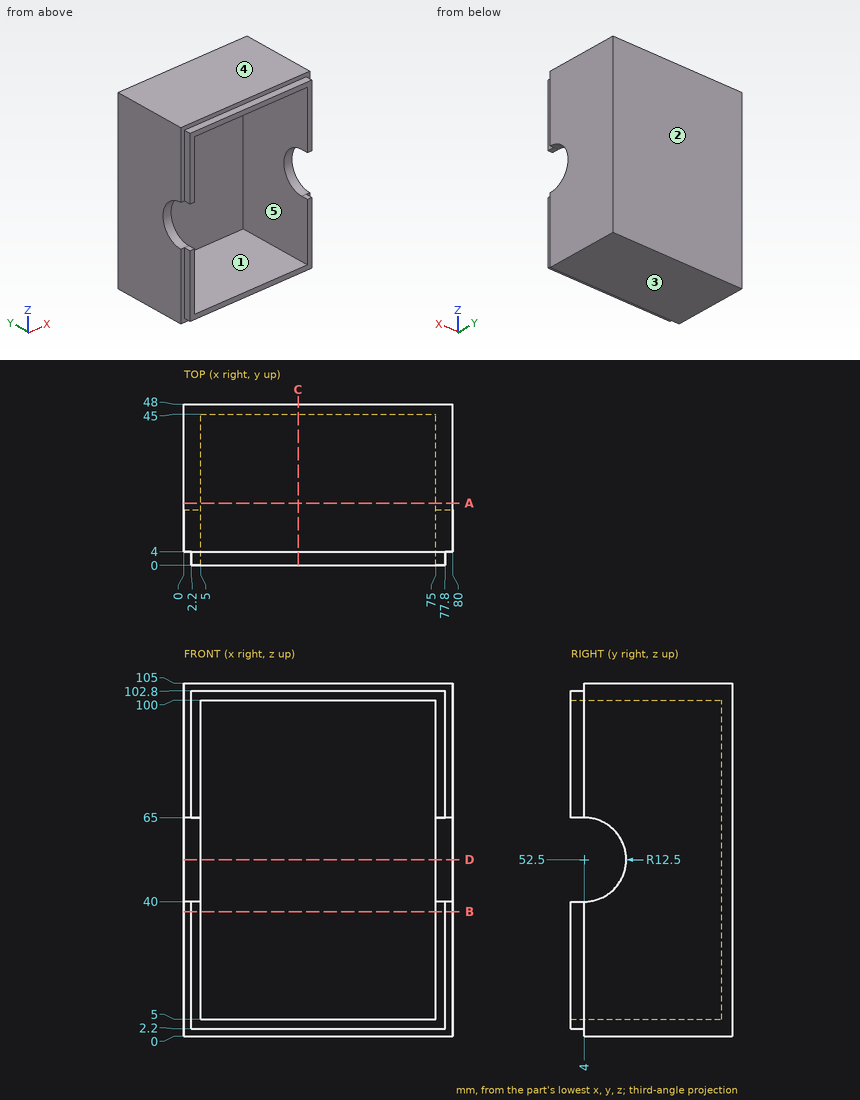
Can you work these out from the drawing? Everything is in mm from the part's minimum corner. A direction names the side the tool comes from. Round coordinates to 2 decimals unless told otherwise and drop trailing zeros. Order: outer loops, then holes, each group sorted by start corner. A loop starts at its lowest first (then second) coordinate and runs counter-clockwise, first axis right, second up. Notation, with made-up numbers: (77, 1.25) -> (135, 1.25) arc R20 ccw to (135, 9.25) -> close; hole circle Ø7 at (-23.5, 40.25). An arc over 180 degrees is marked (long way). Return JSON: item names as keys, results as strings. Group by question number.
1. We'd pull the mould along Z, two halves only. Please class the marked faces 1, 2 and 3: released by +Z, released by -Z, zero draft, split by the parting line, or undercut.
2. Which directions (+Z, -Z, +X, -X, +Y, -Y) give clear straight access to the entire face, cutting with the end or side of a thin tool? Please do the marked faces 4 and 5.
3. If we section it at C-C, the plane x = 34: Write out the boundary of the cut face in (y, z), then the cut area to 3 significant figures.
4. I need wall thicknesses on line 1 (Z direction, x = 46, y = 40.5); line 2 (X direction, y = 41, z = 81.5); line 3 (Y direction, x = 38.5, z = 79). Which ranges of each line are inside material? Lowest first, please. Write a range as [from, to].
5. If we section it at D-D, the plane z = 52.5: Write out the boundary of the cut face in (x, y), then the cut area to 3 significant figures.
6. If we section it at B-B, the plane z = 37: Write out the boundary of the cut face in (x, y), then the cut area to 3 significant figures.
7. Will these pins go through, and if not, where does the flat tip stop? pin 1 (12 mm diameter, centred on x = 52, z = 25.5, fed in from -Y); pin 2 (3 mm diameter, centred on y = 1, z = 82, fed in from +X); pin 3 (2 mm diameter, centred on x = 76, y = 1.5, fed in from -Z).
8. If we section it at A-A, the plane y = 18.5: Write out the boundary of the cut face in (x, z).
Output values:
{
 "1": {"face 1": "undercut", "face 2": "zero draft", "face 3": "released by -Z"},
 "2": {"face 4": "+Z, +X, -X, +Y, -Y", "face 5": "-Y"},
 "3": {"outline": "(0, 2.2) -> (4, 2.2) -> (4, 0) -> (48, 0) -> (48, 105) -> (4, 105) -> (4, 102.8) -> (0, 102.8) -> (0, 100) -> (45, 100) -> (45, 5) -> (0, 5) -> close", "area": "747 mm²"},
 "4": {"line 1": "[0, 5], [100, 105]", "line 2": "[0, 5], [75, 80]", "line 3": "[45, 48]"},
 "5": {"outline": "(0, 16.5) -> (5, 16.5) -> (5, 45) -> (75, 45) -> (75, 16.5) -> (80, 16.5) -> (80, 48) -> (0, 48) -> close", "area": "525 mm²"},
 "6": {"outline": "(0, 4) -> (2.2, 4) -> (2.2, 0) -> (5, 0) -> (5, 45) -> (75, 45) -> (75, 0) -> (77.8, 0) -> (77.8, 4) -> (80, 4) -> (80, 48) -> (0, 48) -> close", "area": "672 mm²"},
 "7": {"pin 1": "y = 45", "pin 2": "x = 77.8", "pin 3": "z = 2.2"},
 "8": {"outline": "(0, 0) -> (80, 0) -> (80, 105) -> (0, 105) -> close; hole (5, 5) -> (75, 5) -> (75, 100) -> (5, 100) -> close"}
}
